```python
from build123d import *

# Parameters (mm, degrees)
SKETCH1_W           = 70
SKETCH1_H           = 50
BOSS_EXTRUDE1_DEPTH = 6
CUT_EXTRUDE1_DEPTH  = 44.428101501


with BuildPart() as part:
    # Sketch1 → Boss-Extrude1 (new body)
    with BuildSketch(Plane.XY):
        Rectangle(SKETCH1_W, SKETCH1_H)
    extrude(amount=BOSS_EXTRUDE1_DEPTH)

    # Sketch2 → Cut-Extrude1 (cut, through all)
    with BuildSketch(Plane.XY):
        with BuildLine():
            Line((23.36, 4.097243552), (23.36, 15.902756448))
            ThreePointArc((23.36, 15.902756448), (26.11, 18.652756448), (28.86, 15.902756448))
            Line((28.86, 15.902756448), (28.86, 4.097243552))
            ThreePointArc((28.86, 4.097243552), (26.11, 1.347243552), (23.36, 4.097243552))
        make_face()
        with BuildLine():
            Line((-23.36, 4.097243552), (-23.36, 15.902756448))
            ThreePointArc((-23.36, 15.902756448), (-26.11, 18.652756448), (-28.86, 15.902756448))
            Line((-28.86, 15.902756448), (-28.86, 4.097243552))
            ThreePointArc((-28.86, 4.097243552), (-26.11, 1.347243552), (-23.36, 4.097243552))
        make_face()
    extrude(amount=CUT_EXTRUDE1_DEPTH, mode=Mode.SUBTRACT)


solid = part.part
```
Work out the finished part from the listing and answer in its coordinate system (mm). A direction names the side the tool comes from. Coordinates: 2 decimals unless noted, no trailing zeros. Order: outer loops, then holes, each group sorted by start corner. A loop starts at its lowest first (then second) coordinate and runs counter-clockwise, first axis right, second up. Notation, with made-up numbers: M 10,36 L 56,36 A7 ccw 56,41 Z; hole C -15,-4 d5. An arc over 180 degrees is marked long. Use CSV: the item, a comma, the result in double quotes.
1) Section C-C on y = 9 is taken. Write down the section's boundary in (x, z).
Worked out:
outline,"M -35,0 L -28.86,0 L -28.86,6 L -35,6 Z; M -23.36,0 L 23.36,0 L 23.36,6 L -23.36,6 Z; M 28.86,0 L 35,0 L 35,6 L 28.86,6 Z"
2) For faces 4 (the face through (26.17, 1.348, 2.958)), 5 (the face through (0, 25, 3)), determine the directions among +Z, -Z, +X, -X, +Y, -Y from which every point of the face is accessible in a straight line to the end or side of a thin tool.
Worked out:
face 4,"+Z, -Z"
face 5,"+Z, -Z, +X, -X, +Y"
3) A flat-ended cylindrical pin translates along its axis: pin 1 Ø1 at (x, y) = (-24, 11) entering from +Z. Find the tip coordinate at first contact, or state that the pin passes through.
Worked out:
pin 1,"passes through"
4) Section B-B on z = 1.6 is taken. Write down the section's boundary in (x, y), plus the area to 3 significant figures.
Worked out:
outline,"M -35,-25 L 35,-25 L 35,25 L -35,25 Z; hole M -28.86,4.1 A2.75 ccw -23.36,4.1 L -23.36,15.9 A2.75 ccw -28.86,15.9 Z; hole M 23.36,4.1 A2.75 ccw 28.86,4.1 L 28.86,15.9 A2.75 ccw 23.36,15.9 Z"
area,"3,320 mm^2"
5) Determine the mould class of faces 1 (the face through (35, 0, 3)), 2 (the face through (-26.17, 1.348, 2.958)), 3 (the face through (0, 0, 0)) for opening direction X: released by +X, released by -X, zero draft, split by the parting line, or undercut.
Worked out:
face 1,"released by +X"
face 2,"undercut"
face 3,"zero draft"
6) Consider line 1 (X direction, y = 8, z = 1.2); line 2 (X direction, y = 2.5, z = 4.15); line 3 (Y direction, x = 26.5, z = 2). Determine where each line is inside the solid, lowest interval first. Write a range as [from, to].
Worked out:
line 1,"x = [-35, -28.86], [-23.36, 23.36], [28.86, 35]"
line 2,"x = [-35, -28.35], [-23.87, 23.87], [28.35, 35]"
line 3,"y = [-25, 1.38], [18.62, 25]"
7) Section A-A on x = 26.11 is taken. Write down the section's boundary in (y, z).
Worked out:
outline,"M -25,0 L 1.35,0 L 1.35,6 L -25,6 Z; M 18.65,0 L 25,0 L 25,6 L 18.65,6 Z"
